```python
from build123d import *

# Parameters (mm, degrees)
FILLET2_R = 0.5
FILLET3_R = 0.5


with BuildPart() as part:
    # Sketch1 → Revolve1 (revolve)
    with BuildSketch(Plane(origin=(0, 0, 0), x_dir=(0, 0, -1), z_dir=(1, 0, 0))):
        Polygon((-12, -7.5), (-8.75, -7.5), (-8.75, -7.15), (-7.65, -7.15), (-7.65, -7.5), (0, -7.5), (0, -4), (-12, -4), align=None)
    revolve1 = revolve(axis=Axis((0, 0, 1000), (0, 0, -1)))

    # Fillet2
    fillet2_edges = [part.edges().sort_by_distance(p)[0] for p in [
        (0, 7.5, 12),
    ]]
    fillet(fillet2_edges, radius=FILLET2_R)

    # Mirror2: Revolve1 across plane
    add(revolve1.mirror(Plane(origin=(0, -4, 0), x_dir=(1, 0, 0), z_dir=(0, 0, -1))))

    # Fillet3
    fillet3_edges = [part.edges().sort_by_distance(p)[0] for p in [
        (0, 7.5, -12),
    ]]
    fillet(fillet3_edges, radius=FILLET3_R)


solid = part.part
```
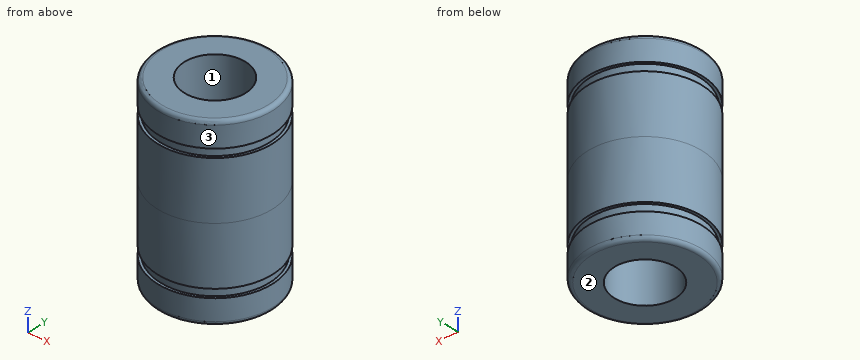
Read the model definition and answer for the solid it produces. Units are mm, in the model's axes. Face numbers are marked on the shaded views. Coordinates: 2 decimals unless noted, no trailing zeros. Loops run counter-clockwise (first coordinate to the right, second up) from the corner with the lowest first, then second, coordinate; pieces in that order, holes last.
(1) The part is cut by section A-A (x = 0). Determine the outline of the cut face in (y, z), and give its area (3 significant figures).
Solution:
outline: (-7.5, -11.5) arc R0.5 ccw to (-7, -12) - (-4, -12) - (-4, 12) - (-7, 12) arc R0.5 ccw to (-7.5, 11.5) - (-7.5, 8.75) - (-7.15, 8.75) - (-7.15, 7.65) - (-7.5, 7.65) - (-7.5, -7.65) - (-7.15, -7.65) - (-7.15, -8.75) - (-7.5, -8.75) - close; (4, -12) - (7, -12) arc R0.5 ccw to (7.5, -11.5) - (7.5, -8.75) - (7.15, -8.75) - (7.15, -7.65) - (7.5, -7.65) - (7.5, 7.65) - (7.15, 7.65) - (7.15, 8.75) - (7.5, 8.75) - (7.5, 11.5) arc R0.5 ccw to (7, 12) - (4, 12) - close
area: 166 mm2
(2) The mould has two halves that part along Y. Classify the marked faces 1, 2 and 3: released by +Y, released by -Y, zero draft, split by the parting line, or undercut.
Solution:
face 1: undercut
face 2: zero draft
face 3: split by the parting line
(3) Flat-ended cylindrical pins translate along their axes: pin 1 Ø8 at (x, z) = (4.5, -5) entering from +Y; pin 2 Ø7.5 at (x, y) = (-3.5, 1) entering from +Z; pin 3 Ø3 at (x, z) = (3, 6) entering from -Y; pin 4 Ø2 at (y, z) = (-3.5, 4.5) entering from +X. Find the tip coordinate at first contact, or state that the pin passes through.
Solution:
pin 1: stops at y = 7.48
pin 2: stops at z = 12
pin 3: stops at y = -7.35
pin 4: stops at x = 7.07
(4) The part is cut by section C-C (z = -5). Determine the outline of the cut face in (x, y).
Solution:
outline: circle Ø15 at (0, 0); hole circle Ø8 at (0, 0)
(5) Consider line 1 along Y through (x, z) = (0, -0.75); line 2 along Z through (x, y) = (-5, 5). Determine where each line is inside the solid, lowest interval first.
Solution:
line 1: y = -7.5 to -4, 4 to 7.5
line 2: z = -11.99 to 11.99
